```python
from build123d import *

# Parameters (mm, degrees)
F0_W     = 110
F0_H     = 125
F0_W_2   = 100
F0_H_2   = 105
F1_DEPTH = 150
F2_W     = 4
F2_H     = 4
F3_DEPTH = 150


# Not quite as in the source:
# - a pattern or mirror of a feature is missing from the dataset's text; its kind, count and spacing are read off the source's solid


with BuildPart() as f1:
    # F0 (on Front) → F1 (new body)
    with BuildSketch(Plane.XZ):
        Rectangle(F0_W, F0_H)
        Rectangle(F0_W_2, F0_H_2, mode=Mode.SUBTRACT)
    extrude(amount=F1_DEPTH)

    # F2 (on face) → F3 (cut, through all)
    with BuildSketch(Plane.XZ.offset(150)):
        with Locations((-42, 54.5)):
            Rectangle(F2_W, F2_H)
        with Locations((-38, 54.5)):
            Rectangle(F2_W, F2_H)
        with Locations((-3, 54.5)):
            Rectangle(F2_W, F2_H)
        with Locations((-7, 54.5)):
            Rectangle(F2_W, F2_H)
        with Locations((32, 54.5)):
            Rectangle(F2_W, F2_H)
        with Locations((28, 54.5)):
            Rectangle(F2_W, F2_H)
    f3 = extrude(amount=-F3_DEPTH, mode=Mode.SUBTRACT)

    # F3_copies: F3 across plane
    add(f3.mirror(Plane(origin=(0, 0, 0), x_dir=(-1, 0, 0), z_dir=(0, 0, -1))), mode=Mode.SUBTRACT)


solid = f1.part
```
Source: CAD feature listing. Evaluate the final solid. Frame: model axes, mm. A direction names the side the tool comes from. Round coordinates to 2 decimals unless told otherwise and drop trailing zeros. Loops run counter-clockwise (first coordinate to the right, second up) from the corner with the lowest first, then second, coordinate; pieces in that order, holes last. Notation, with made-up numbers: M 17,79 L 58,79 A15 ccw 58,83 Z; hole C 45,25 d4. An arc over 180 degrees is marked long. Use a Markdown table: item, result. Add a question column.
1. Section query C-C on z = 38. Return the cut outline in (x, y), then the cut area to 3 significant figures.
2. Mould query, pull axis X, two halves, no side actions, for faces 3 (the flat face through (-55, -74, -1)), 4 (the flat face through (-23, -74, 52.5)), 5 (the flat face through (0, 0, 56)). Classes: pulls with the +X half, pulls with the -X half, needs draft (parallel to the pull), parting line crosses it, or undercut.
3. Line query: line 1 (Z direction, x = 17, y = -123); line 2 (X direction, y = -24.5, z = -11.5); line 3 (X direction, y = -76.5, z = -55.5). Output: solid intervals per line, ascending.
4. Reachability of faces 1 (the flat face through (0, -150, 56)), 2 (the flat face through (-1, -76, 54)) from +Z, -Z, +X, -X, +Y, -Y: full face, straight path, thin tool, end or side. Return the list, or none.
5. Section query A-A on x = 31. Return the cut outline in (y, z).
Reported:
| question | item | result |
|---|---|---|
| 1 | outline | M -55,-150 L -50,-150 L -50,0 L -55,0 Z; M 50,-150 L 55,-150 L 55,0 L 50,0 Z |
| 1 | area | 1,500 mm² |
| 2 | face 3 | pulls with the -X half |
| 2 | face 4 | undercut |
| 2 | face 5 | needs draft |
| 3 | line 1 | z = -62.5 to -52.5, 52.5 to 62.5 |
| 3 | line 2 | x = -55 to -50, 50 to 55 |
| 3 | line 3 | x = -55 to -44, -36 to -9, -1 to 26, 34 to 55 |
| 4 | face 1 | +Z, -Z, +X, -X, -Y |
| 4 | face 2 | +Y, -Y |
| 5 | outline | M -150,-62.5 L 0,-62.5 L 0,-56.5 L -150,-56.5 Z; M -150,56.5 L 0,56.5 L 0,62.5 L -150,62.5 Z |
